Geometry check sheet. Reference: the model listing, model coordinates, mm. Face numbers are marked on the shaded views. A direction names the side the tool comes from. Round coordinates to 2 decimals unless told otherwise and drop trailing zeros. Write each loop counter-clockwise with the first axis right and the second up, starting at its lowest first coordinate (ties: lowest second). Pieces come first, ordered by that corner, then holes. Notation, with made-up numbers: M 52.25,-18.75 L 81.25,-18.75 A21 cw 81.25,-8.75 Z; hole C -32.5,51.25 d4. An arc over 180 degrees is marked long. Put each result on its own line as item: value. Start each with the question number.
(1) Section check D-D on z = -17. Record the cut outline in (x, y).
(2) Section check B-B on x = 16.25. Record the cut outline in (y, z), then the cut area to 3 significant figures.
(3) Gauge pin test, flat ends, axial feed: pin 1 (1.5 mm diameter, centred on y = 14, z = -69, fed in from -X); pin 2 (8 mm diameter, centred on x = 20.5, z = -8, fed in from +Y); pin 3 (5 mm diameter, centred on x = 21, z = -47, fed in from +Y); pin 4 (4 mm diameter, centred on x = 3, z = -47, fed in from +Y). Record the tip position at first contact, or that the pin passes through.
(4) Mould release check, pull along Y, two halves, no side actions. Record for the marked faces 1, 2 and 3: pulls with the +Y half, pulls with the -Y half, needs draft (parallel to the pull), parting line crosses it, or undercut.
(5) Tool access check on the marked faces 4, 5 and 6. Record the directions out of +Z, -Z, +X, -X, +Y, -Y that give a thin tool (end or side, any length) a straight path to the whole face; none if there is none.
(6) Material ranges on probe 1 along Y at (x, z) = (1.75, -31.5); probe 2 along Z at (x, y) = (12.25, 33.5); probe 3 along Z at (x, y) = (18.5, 46), recorded low to high.
(7) Section check A-A on y = 29.5. Record the cut outline in (x, z), then the cut area to 3 significant figures.
(8) Section check C-C on z = -54. Record the cut outline in (x, y).
from build123d import *

# Parameters (mm, degrees)
SKETCH1_W           = 28
SKETCH1_H           = 78
BOSS_EXTRUDE1_DEPTH = 58
CUT_EXTRUDE1_START  = -28
CUT_EXTRUDE1_DEPTH  = 28
CUT_EXTRUDE2_DEPTH  = 10
SKETCH3_R           = 3
BOSS_EXTRUDE2_DEPTH = 6


# Read off the part's stored shape, not the designer's step: Cut-Extrude1
with BuildPart() as part:
    # Sketch1 → Boss-Extrude1 (new body)
    with BuildSketch(Plane(origin=(0, 0, 0), x_dir=(1, 0, 0), z_dir=(0, 1, 0))):
        with Locations((14, 39)):
            Rectangle(SKETCH1_W, SKETCH1_H)
    extrude(amount=BOSS_EXTRUDE1_DEPTH)

    # Cut-Extrude1 outline → Cut-Extrude1 (cut)
    with BuildSketch(Plane(origin=(28, 0, 0), x_dir=(0, 0, -1), z_dir=(1, 0, 0)).offset(CUT_EXTRUDE1_START)):
        Polygon((24, 16), (24, 34), (40, 34), (51.191383796, 58), (0, 58), (0, 16), align=None)
        Polygon((78, 58), (51.191383796, 58), (64.786000601, 51.660726074), (47.998924908, 15.660726074), (52.530463843, 13.547634765), (69.317539536, 49.547634765), (78, 45.498936959), align=None)
    extrude(amount=CUT_EXTRUDE1_DEPTH, mode=Mode.SUBTRACT)

    # Sketch2_3 → Cut-Extrude2 (cut)
    with BuildSketch(Plane(origin=(28, 0, 0), x_dir=(0, 0, -1), z_dir=(1, 0, 0))):
        Polygon((0, 16), (0, 8), (27.876000888, 8), (40, 34), (24, 34), (24, 16), align=None)
    extrude(amount=-CUT_EXTRUDE2_DEPTH, mode=Mode.SUBTRACT)

    # Sketch3 → Boss-Extrude2 (add)
    with BuildSketch(Plane(origin=(0, 67.248278227, -31.358387135), x_dir=(1, 0, 0), z_dir=(0, 0.906307787036651, -0.4226182617406971))):
        with Locations(Location((7, 29.383290582, 0), (0, 0, 90))):
            Circle(SKETCH3_R)
        with Locations(Location((21, 29.383290582, 0), (0, 0, 90))):
            Circle(SKETCH3_R)
    extrude(amount=BOSS_EXTRUDE2_DEPTH)


solid = part.part
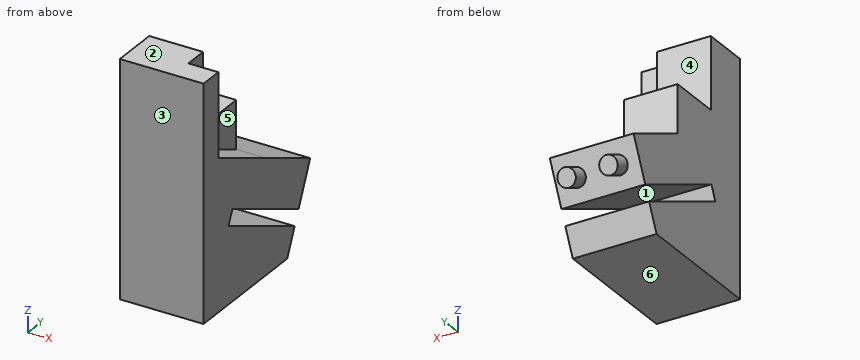
Answers follow:
1. outline: M 0,0 L 28,0 L 28,8 L 18,8 L 18,16 L 0,16 Z
2. outline: M 0,-78 L 45.5,-78 L 49.55,-69.32 L 13.55,-52.53 L 15.66,-48 L 51.66,-64.79 L 58,-51.19 L 34,-40 L 34,-24 L 16,-24 L 16,0 L 0,0 Z
2. area: 2,630 mm^2
3. pin 1: stops at x = 0
3. pin 2: stops at y = 16
3. pin 3: stops at y = 54.37
3. pin 4: stops at y = 53.3
4. face 1: undercut
4. face 2: needs draft
4. face 3: pulls with the -Y half
5. face 4: +Z, +X, -X, +Y
5. face 5: +Z, +X, +Y
5. face 6: -Z, +X, -X, +Y, -Y
6. probe 1: y = 0 to 34
6. probe 2: z = -78 to -61.83, -56.32 to -24
6. probe 3: z = -76.93 to -67.66, -62.15 to -45.6
7. outline: M 0,-78 L 28,-78 L 28,-59.97 L 0,-59.97 Z; M 0,-54.45 L 28,-54.45 L 28,-37.9 L 18,-37.9 L 18,-24 L 0,-24 Z
7. area: 1,220 mm^2
8. outline: M 0,0 L 28,0 L 28,16.7 L 0,16.7 Z; M 0,28.53 L 28,28.53 L 28,56.69 L 0,56.69 Z
